from build123d import *

# Parameters (mm, degrees)
SKETCH1_R           = 24
BOSS_EXTRUDE1_DEPTH = 200
SKETCH2_R           = 15
BOSS_EXTRUDE2_DEPTH = 40
LPATTERN1_COUNT     = 2
LPATTERN1_PITCH     = 240


with BuildPart() as part:
    # Sketch1 → Boss-Extrude1 (new body)
    with BuildSketch(Plane.XY):
        Circle(SKETCH1_R)
    extrude(amount=BOSS_EXTRUDE1_DEPTH)

    # Sketch2 → Boss-Extrude2 (add)
    with BuildSketch(Plane(origin=(0, 0, 0), x_dir=(-1, 0, 0), z_dir=(0, 0, -1))):
        Circle(SKETCH2_R)
    boss_extrude2 = extrude(amount=BOSS_EXTRUDE2_DEPTH)

    # LPattern1: Boss-Extrude2 ×2
    with Locations(*[(0, 0, i * LPATTERN1_PITCH) for i in range(1, LPATTERN1_COUNT)]):
        add(boss_extrude2)


solid = part.part
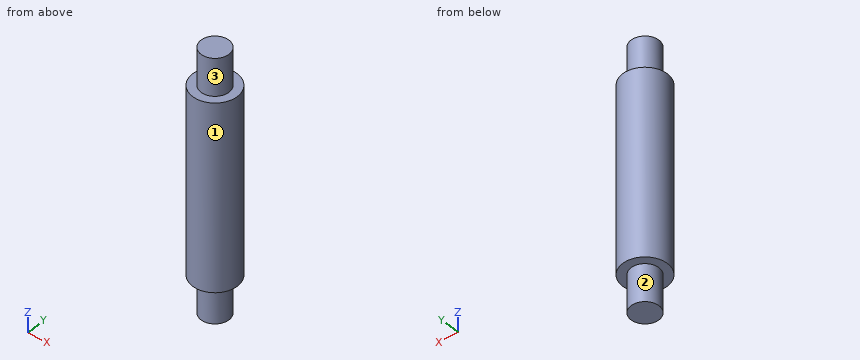
Can you work these out from the model? Positions are in its coordinate system, mm. Face numbers are marked on the shaded views. A direction names the side the tool comes from. Round coordinates to 2 decimals unless told otherwise and drop trailing zeros. Order: outer loops, then holes, each group sorted by start corner. A loop starts at its lowest first (then second) coordinate and runs counter-clockwise, first axis right, second up. Notation, with made-up numbers: (81.5, 54) - (93.5, 54) arc R18 cw to (93.5, 68) - close; hole circle Ø10 at (51.5, 61.25). An arc over 180 degrees is marked (long way). Answer in a Markdown table with one row per item.
(1) Please list where these lines run through material, in increasing order: L1, parallel to Z at x = -8, y = -20; L2, parallel to Y at x = 1, z = 135; L3, parallel to Y at x = 21, z = 10. Write a range as from..to.
From the geometry:
| item | result |
|---|---|
| L1 | z = 0..200 |
| L2 | y = -23.98..23.98 |
| L3 | y = -11.62..11.62 |
(2) For P1, Ø5, axis at y = 10, z = 157.5, coming from the -X side; P2, Ø8, axis at x = -9, z = 169.5, coming from the -Y side; P3, Ø12, axis at y = -9.5, z = 199.5, coming from the +X side, each with a flat end and sliding along its axis, tell me the tip position at first contact or that it passes through.
From the geometry:
| item | result |
|---|---|
| P1 | stops at x = -22.8 |
| P2 | stops at y = -23.47 |
| P3 | stops at x = 23.74 |
(3) Suppose I cut it at A-A, the plane y = 0. Please give me the cut outline in (x, z), plus the area to 3 significant figures.
From the geometry:
| item | result |
|---|---|
| outline | (-24, 0) - (-15, 0) - (-15, -40) - (15, -40) - (15, 0) - (24, 0) - (24, 200) - (15, 200) - (15, 240) - (-15, 240) - (-15, 200) - (-24, 200) - close |
| area | 12,000 mm2 |
(4) Suppose I cut it at C-C, the plane z = 45. Please give me the cut outline in (x, y).
From the geometry:
| item | result |
|---|---|
| outline | circle Ø48 at (0, 0) |
(5) Suppose I cut it at D-D, the plane z = 203.5. Please give me the cut outline in (x, y), plus the area to 3 significant figures.
From the geometry:
| item | result |
|---|---|
| outline | circle Ø30 at (0, 0) |
| area | 707 mm2 |
(6) Which directions (+Z, -Z, +X, -X, +Y, -Y) give clear straight access to the entire face, cutting with the end or side of a thin tool? Please do the marked faces 1, 2 and 3.
From the geometry:
| item | result |
|---|---|
| face 1 | +Z, -Z |
| face 2 | -Z |
| face 3 | +Z |
